from build123d import *

# Parameters (mm, degrees)
SKETCH2_R           = 25
BOSS_EXTRUDE1_DEPTH = 10
FILLET1_R           = 3
SKETCH3_W           = 28.25
SKETCH3_H           = 28.25
BOSS_EXTRUDE2_DEPTH = 1


with BuildPart() as part:
    # Sketch2 → Boss-Extrude1 (new body)
    with BuildSketch(Plane(origin=(0, 0, 0), x_dir=(1, 0, 0), z_dir=(0, 1, 0))):
        with Locations(Location((0, 0, 0), (0, 0, 270))):
            Circle(SKETCH2_R)
    extrude(amount=BOSS_EXTRUDE1_DEPTH)

    # Fillet1
    fillet1_edges = [part.edges().sort_by_distance(p)[0] for p in [
        (0, 0, -25),
        (0, 10, -25),
    ]]
    fillet(fillet1_edges, radius=FILLET1_R)

    # Sketch3 → Boss-Extrude2 (add)
    with BuildSketch(Plane(origin=(0, 0, 0), x_dir=(-1, 0, 0), z_dir=(0, -1, 0))):
        Rectangle(SKETCH3_W, SKETCH3_H)
    extrude(amount=BOSS_EXTRUDE2_DEPTH)


solid = part.part
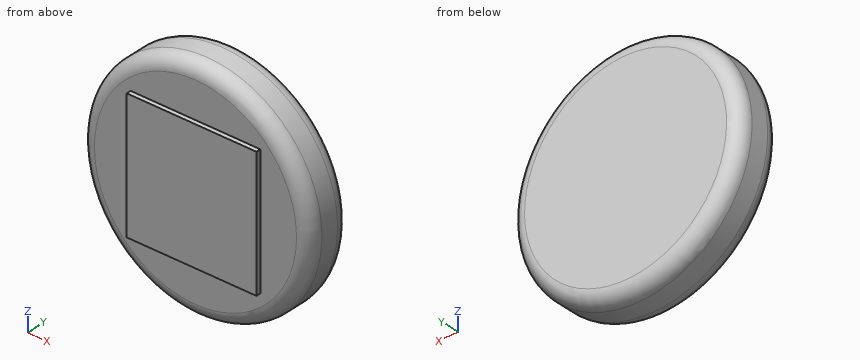
Verification items for the finished model (mm, model axes). Coordinates: 2 decimals unless noted, no trailing zeros. Loops run counter-clockwise (first coordinate to the right, second up) from the corner with the lowest first, then second, coordinate; pieces in that order, holes last. Notation, with made-up numbers: M 32,55.5 L 62,55.5 A31 ccw 62,93.5 Z; hole C 68.25,-26 d5. An arc over 180 degrees is marked long. One line per item, written item: value.
1. Section check B-B on x = 0. Record the cut outline in (y, z) (3 decimals), plus the area to 3 significant figures.
Answers follow:
outline: M -1,-14.125 L 0,-14.125 L 0,-22 A3 ccw 3,-25 L 7,-25 A3 ccw 10,-22 L 10,22 A3 ccw 7,25 L 3,25 A3 ccw 0,22 L 0,14.125 L -1,14.125 Z
area: 521 mm^2
2. Section check A-A on z = 0. Record the cut outline in (x, y) (3 decimals).
Answers follow:
outline: M -25,3 A3 ccw -22,0 L -14.125,0 L -14.125,-1 L 14.125,-1 L 14.125,0 L 22,0 A3 ccw 25,3 L 25,7 A3 ccw 22,10 L -22,10 A3 ccw -25,7 Z
3. Section check C-C on y = 5.25. Record the cut outline in (x, z), plus the area to 3 significant figures.
Answers follow:
outline: C 0,0 d50
area: 1,960 mm^2
4. Gauge pin test, flat ends, axial feed: P1, Ø0.5, axis at x = -3, y = -0.5, coming from the +Z side (3 decimals); P2, Ø2, axis at x = -10.5, y = 4.5, coming from the -Z side; P3, Ø1, axis at y = 8.5, z = 7.5, coming from the +X side. Record the tip position at first contact, or that the pin passes through.
Answers follow:
P1: z = 14.125
P2: z = -23.12
P3: x = 23.72
5. Material ranges on line 1 along Y through (x, z) = (-16, -11); line 2 along X through (y, z) = (5, 0); line 3 along Z through (x, y) = (18, 4.25), recorded low to high. Write a range as from..to.
Answers follow:
line 1: 0..10
line 2: -25..25
line 3: -17.35..17.35
